Verification items for this drawing (mm, ordinates from the low corner). A direction names the side the tool comes from. Round coordinates to 2 decimals unless told otherwise and drop trailing zeros. Write each loop counter-clockwise with the first axis right and the second up, starting at its lowest first coordinate (ties: lowest second). Pieces come first, ordered by that corner, then holes. Notation, with made-up numbers: M 49.25,65 L 95.25,65 A23 cw 95.25,85 Z; hole C -27.75,52.5 d7. An arc over 180 degrees is marked long. Write each question's results on one line, items separated by ' | '.
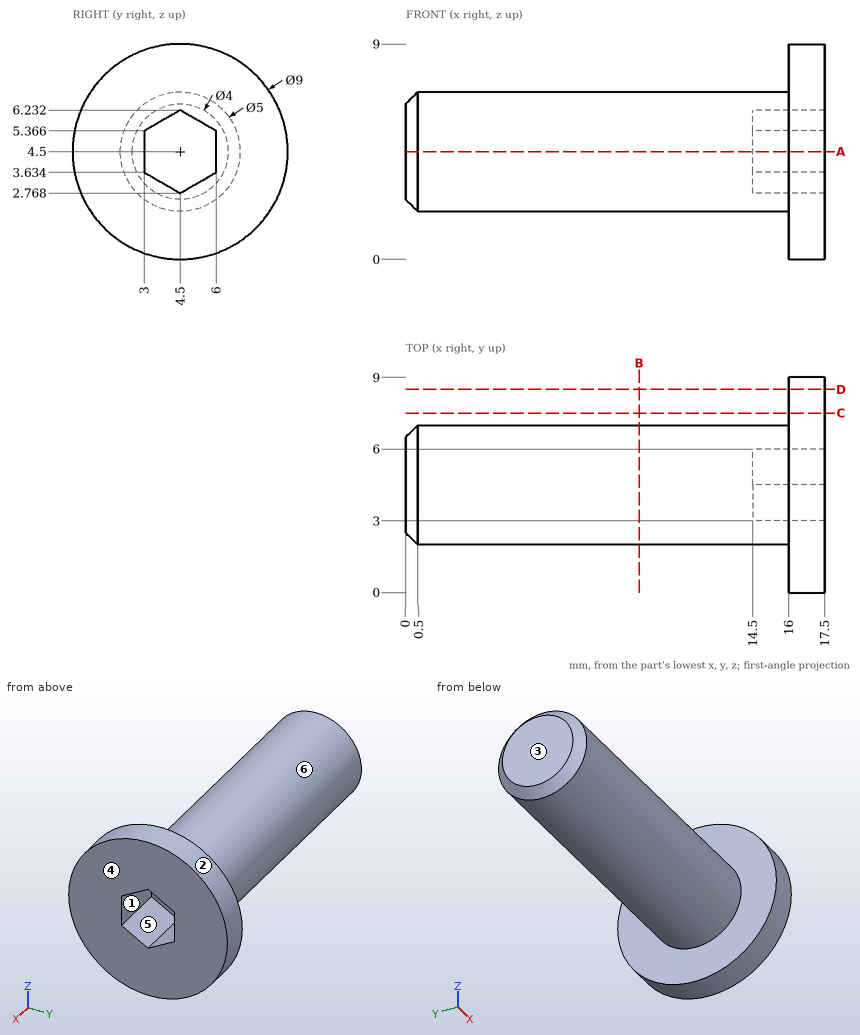
1) Sectioned sample at C-C, the plane y = 7.5. Record the cut outline in (x, z).
Calculated:
outline: M 16,1.15 L 17.5,1.15 L 17.5,7.85 L 16,7.85 Z
2) Depth check by flat-ended pin: P1, Ø2, axis at x = 9.5, y = 6.5, coming from the +Z side; P2, Ø0.9, axis at x = 15.5, z = 4.5, coming from the -Y side; P3, Ø2, axis at x = 8.5, y = 2.5, coming from the -Z side. Enter the tip coordinate at first touch or a pass-through.
Calculated:
P1: stops at z = 6.79 | P2: stops at y = 2 | P3: stops at z = 2.21
3) Material ranges on line 1 (Y direction, x = 7, z = 6); line 2 (X direction, y = 7.25, z = 8), recorded low to high. Write a range as [from, to].
Calculated:
line 1: y = [2.5, 6.5] | line 2: x = [16, 17.5]
4) Access from +Z, -Z, +X, -X, +Y, -Y to the whole of each face (thin tool, end or side, straight path). Record for the marked faces 4, 5 and 6.
Calculated:
face 4: +Z, -Z, +X, +Y, -Y | face 5: +X | face 6: -X
5) Draft check along Z on the marked faces 1, 2 and 3. Enter one of: pulls with the +Z half, pulls with the -Z half, needs draft (parallel to the pull), parting line crosses it, or undercut.
Calculated:
face 1: undercut | face 2: parting line crosses it | face 3: needs draft
6) Sectioned sample at B-B, the plane x = 9.75. Record the cut outline in (y, z), and give its area (3 significant figures).
Calculated:
outline: C 4.5,4.5 d5 | area: 19.6 mm²
7) Sectioned sample at A-A, the plane z = 4.5. Record the cut outline in (x, y).
Calculated:
outline: M 0,2.5 L 0.5,2 L 16,2 L 16,0 L 17.5,0 L 17.5,3 L 14.5,3 L 14.5,6 L 17.5,6 L 17.5,9 L 16,9 L 16,7 L 0.5,7 L 0,6.5 Z
8) Sectioned sample at D-D, the plane y = 8.5. Record the cut outline in (x, z).
Calculated:
outline: M 16,2.44 L 17.5,2.44 L 17.5,6.56 L 16,6.56 Z
